Autodesk Inventor part; units mm, degrees
ref_plane "YZ Plane" through (0, 0, 0) normal (1, 0, 0) x (0, 1, 0)
ref_plane "XZ Plane" through (0, 0, 0) normal (0, 1, 0) x (-1, 0, 0)
ref_plane "XY Plane" through (0, 0, 0) normal (0, 0, 1) x (1, 0, 0)
sketch "Sketch1" plane through (0, 0, 0) normal (0, 0, 1) x (1, 0, 0)
  line L0 (0, 0) -> (68.58, 0)
  line L1 (68.58, 0) -> (68.58, 46.228)
  line L2 (68.58, 46.228) -> (0, 46.228)
  line L3 (0, 46.228) -> (0, 0)
  dimension "d0" = 68.58
  dimension "d1" = 46.228
extrude "Extrusion1" add sketch "Sketch1" along normal blind 2.54
sketch "Sketch2" plane through (0, 0, 2.54) normal (0, 0, 1) x (1, 0, 0)
  line L0 (0, 46.228) -> (0, 0)
  line L1 (0, 46.228) -> (68.58, 46.228)
  line L2 (68.58, 46.228) -> (68.58, 0)
  line L3 (68.58, 0) -> (0, 0)
  line L4 (0, 0) -> (0, 46.228)
  line L5 (6.35, 43.688) -> (59.69, 43.688)
  line L6 (59.69, 43.688) -> (59.69, 28.448)
  line L7 (59.69, 28.448) -> (6.35, 28.448)
  line L8 (6.35, 28.448) -> (6.35, 43.688)
  line L9 (3.048, 28.448) -> (65.532, 28.448)
  line L10 (65.532, 28.448) -> (65.532, 3.048)
  line L11 (65.532, 3.048) -> (3.048, 3.048)
  line L12 (3.048, 3.048) -> (3.048, 28.448)
  dimension "d4" = 62.484
  dimension "d5" = 53.34
  dimension "d6" = 15.24
  dimension "d7" = 25.4
  dimension "d8" = 3.048
  dimension "d9" = 3.048
  dimension "d10" = 0
  dimension "d13" = 6.35
extrude "Extrusion2" [suppressed]
chamfer "Chamfer1" [suppressed]
chamfer "Chamfer2" [suppressed]
sketch "Sketch3" plane through (0, 0, 2.54) normal (0, 0, 1) x (1, 0, 0)
  circle A0 centre (34.29, 36.068) radius 3.4925
  line L0 (0, 0) -> (68.58, 0)
  line L1 (0, 46.228) -> (0, 0)
  line L2 (68.58, 46.228) -> (0, 46.228)
  line L3 (68.58, 0) -> (68.58, 46.228)
  dimension "d22" = 10.16
  dimension "d23" = 34.29
  dimension "d24" = 6.985
extrude "Extrusion3" cut sketch "Sketch3" against normal up to surface (2.54 mm away) contours A0
sketch "Sketch4" plane through (0, 0, 2.54) normal (0, 0, 1) x (1, 0, 0)
  line L0 (59.69, 28.448) -> (59.69, 43.688)
  line L1 (59.69, 43.688) -> (6.35, 43.688)
  circle A0 centre (44.704, 36.068) radius 1.4732
  point P0 (0, 0)
  dimension "d27" = 2.9464
  dimension "d28" = 7.62
  dimension "d29" = 14.986
extrude "Extrusion4" add sketch "Sketch4" along normal blind 7.62
fillet "Fillet1" radius 1.4732 1 edges at (43.2308, 36.068, 10.16)
fillet "Fillet2" radius 2.54 4 edges at (0, 46.228, 1.27) (68.58, 46.228, 1.27) (68.58, 0, 1.27) (0, 0, 1.27)
sketch "Sketch5" plane through (0, 0, 2.54) normal (0, 0, 1) x (1, 0, 0)
  circle A0 centre (34.29, 36.068) radius 3.4925
  line L0 (26.67, 43.688) -> (41.91, 43.688)
  line L1 (41.91, 43.688) -> (41.91, 24.638)
  line L2 (41.91, 24.638) -> (26.67, 24.638)
  line L3 (26.67, 24.638) -> (26.67, 43.688)
  point P0 (0, 0)
  dimension "d34" = 19.05
  dimension "d35" = 15.24
  dimension "d36" = 7.62
  dimension "d37" = 7.62
extrude "Extrusion5" [suppressed]
hole "Hole1" [suppressed]
equation "\"d9\" = d8"
properties part number "Front_Plate"
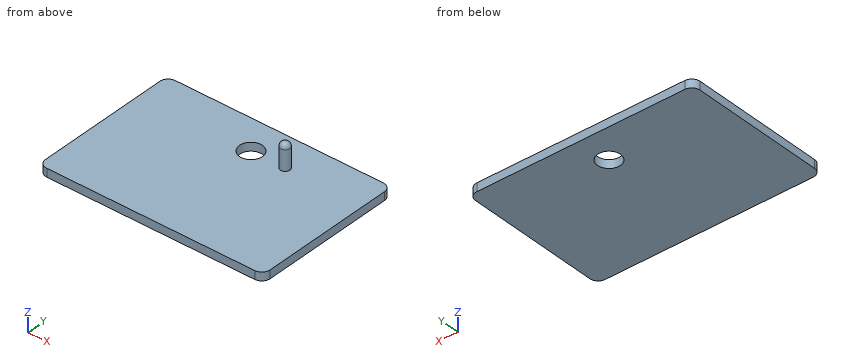
Work out the finished part from the listing and answer in its coordinate system (mm). Give positions to 0.01 mm unless a question says otherwise; leave off trailing zeros. Loops run counter-clockwise (first coordinate to the right, second up) from the corner with the lowest first, then second, coordinate; pieces in that order, holes last. Notation, with made-up numbers: (-4.75, -36.5) -> (19.25, -36.5) arc R7 cw to (19.25, -29.5) -> close; hole circle Ø4 at (15.5, 45). An arc over 180 degrees is marked (long way). Put each result on its own line as item: value. Start each with the question number.
Item 1: The part is cut by section B-B (y = 17). Give the vertices of the cut face in (x, z), then the cut area to 3 significant figures.
Item 2: The part is cut by section C-C (z = 5.25). Give the vertices of the cut face in (x, y), then the cut area to 3 significant figures.
Item 3: The part is cut by section D-D (x = 11.5). Give the vertices of the cut face in (y, z), then the cut area to 3 significant figures.
Item 4: Each of these flat-tipped pins is pushed along its axis until it touches: P1, Ø3, axis at x = 45.5, z = 7, coming from the +Y side; P2, Ø9, axis at x = 34.29, y = 36.068, coming from the +Z side. Where does it stop, or does it pass through?
Item 5: Find the intervals of material crossed by L1, parallel to Y at x = 34.29, z = 0.6; L2, parallel to Z at x = 19, y = 22, in increasing order. Write a range as [from, to].
Item 6: The part is cut by section A-A (x = 34.29). Give the vertices of the cut face in (y, z).
Answers below:
1. outline: (0, 0) -> (68.58, 0) -> (68.58, 2.54) -> (0, 2.54) -> close
1. area: 174 mm2
2. outline: circle Ø2.95 at (44.7, 36.07)
2. area: 6.82 mm2
3. outline: (0, 0) -> (46.23, 0) -> (46.23, 2.54) -> (0, 2.54) -> close
3. area: 117 mm2
4. P1: y = 37.54
4. P2: z = 2.54
5. L1: [0, 32.58], [39.56, 46.23]
5. L2: [0, 2.54]
6. outline: (0, 0) -> (32.58, 0) -> (32.58, 2.54) -> (0, 2.54) -> close; (39.56, 0) -> (46.23, 0) -> (46.23, 2.54) -> (39.56, 2.54) -> close
